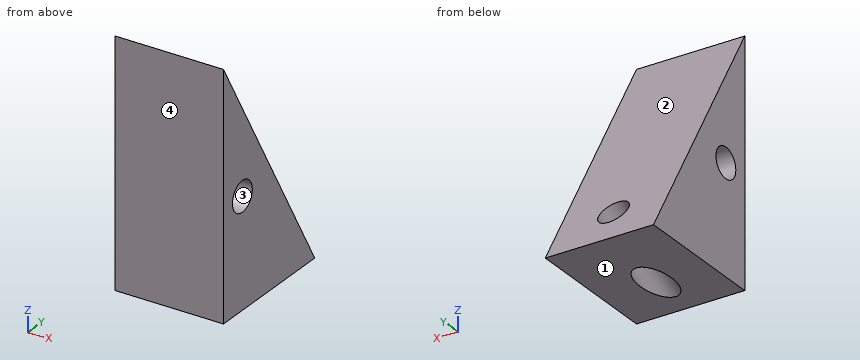
```python
from build123d import *

# Parameters (mm, degrees)
BOSS_EXTRUDE1_DEPTH   = 15
M5X0_8_TAPPED_HOLE1_D = 4.2
M5X0_8_TAPPED_HOLE2_D = 4.2


with BuildPart() as part:
    # Sketch3 → Boss-Extrude1 (new body)
    with BuildSketch(Plane(origin=(0, 0, 0), x_dir=(0, 0, -1), z_dir=(1, 0, 0))):
        Polygon((0, 0), (-33.49045709, 0), (0, 19.335724416), align=None)
    extrude(amount=BOSS_EXTRUDE1_DEPTH)

    # M5x0.8 Tapped Hole1 (through all)
    with Locations(Plane(origin=(15, 0, 0), x_dir=(0, 0, -1), z_dir=(1, 0, 0))):
        with Locations((-15, 4)):
            Hole(M5X0_8_TAPPED_HOLE1_D / 2)

    # M5x0.8 Tapped Hole2 (through all)
    with Locations(Plane(origin=(0, 14.501793312, 8.372614273), x_dir=(1, 0, 0), z_dir=(0, 0.866025404, 0.5))):
        with Locations((7.5, 3.667862208)):
            Hole(M5X0_8_TAPPED_HOLE2_D / 2)


solid = part.part
```
Geometry check sheet. Reference: the model listing, model coordinates, mm. Face numbers are marked on the shaded views. Give positions to 0.01 mm unless a question says otherwise; leave off trailing zeros. Order: outer loops, then holes, each group sorted by start corner. A loop starts at its lowest first (then second) coordinate and runs counter-clockwise, first axis right, second up. Notation, with made-up numbers: (6.5, 70.25) - (62.5, 70.25) arc R29 cw to (62.5, 97.25) - close; hole circle Ø10 at (13, -18). An arc over 180 degrees is marked (long way). Write item = value, one per line. Start each with the question number.
1) Gauge pin test, flat ends, axial feed: pin 1 Ø3 at (x, y) = (8.5, 13.5) entering from -Z; pin 2 Ø1.5 at (x, y) = (12.5, 14) entering from +Z; pin 3 Ø4 at (y, z) = (4, 15) entering from -X; pin 4 Ø1 at (x, y) = (3.5, 8) entering from +Z. Record the tip position at first contact, or that the pin passes through.
2) Section check D-D (x = 4). Enter the section's corners in (y, z), then the cut area to 3 significant figures.
3) Draft check along Z on the marked faces 1, 2, 3 and 4. Enter one of: released by +Z, released by -Z, zero draft, split by the parting line, or undercut.
4) Section check A-A (y = 2.75). Enter the section's corners in (x, z), then the cut area to 3 significant figures.
5) Scan lines: L1, parallel to Z at x = 8.75, y = 4.5; L2, parallel to X at y = 15.5, z = 4.5; L3, parallel to Y at x = 10.25, z = 15. Record each from-to range of solid material in increasing order.
6) Section check C-C (x = 6.75). Enter the section's corners in (y, z), then the cut area to 3 significant figures.
7) Section check B-B (z = 15). Enter the section's corners in (x, y).
Geometry check:
q1.pin_1 = 0
q1.pin_2 = 10.54
q1.pin_3 = through
q1.pin_4 = 20.5
q2.outline = (0, 0) - (19.34, 0) - (0, 33.49) - close; hole circle Ø4.2 at (4, 15)
q2.area = 310 mm2
q3.face_1 = released by -Z
q3.face_2 = released by +Z
q3.face_3 = undercut
q3.face_4 = zero draft
q4.outline = (0, 0) - (15, 0) - (15, 13.31) - (0, 13.31) - close; (0, 16.69) - (15, 16.69) - (15, 28.73) - (0, 28.73) - close
q4.area = 380 mm2
q5.L1 = 0.31 to 12.96, 17.04 to 25.7
q5.L2 = 0 to 5.41, 9.59 to 15
q5.L3 = 0 to 1.9, 6.1 to 10.68
q6.outline = (0, 0) - (3.41, 0) - (15.35, 6.89) - (0, 33.49) - close; (11.26, 0) - (19.34, 0) - (17.32, 3.5) - close; hole circle Ø4.2 at (4, 15)
q6.area = 269 mm2
q7.outline = (0, 0) - (15, 0) - (15, 1.9) - (0, 1.9) - close; (0, 6.1) - (15, 6.1) - (15, 10.68) - (0, 10.68) - close
